Read the model definition and answer for the solid it produces. Units are mm, in the model's axes. Coordinates: 2 decimals unless noted, no trailing zeros. Order: outer loops, then holes, each group sorted by start corner. A loop starts at its lowest first (then second) coordinate and runs counter-clockwise, first axis right, second up. Notation, with made-up numbers: (4.5, 64.5) - (41.5, 64.5) arc R16 cw to (41.5, 83.5) - close; hole circle Ø4 at (6, 50). An arc over 180 degrees is marked (long way). Answer as a JSON object with one key per item and string values. Group by question number.
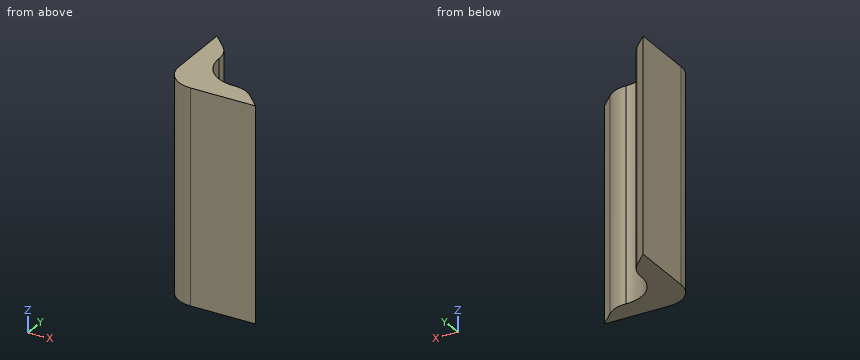
from build123d import *

# Parameters (mm, degrees)
BOSS_EXTRUDE1_DEPTH = 9.525
CHAMFER1_SIZE       = 2
FILLET1_R           = 2.54
FILLET2_R           = 2.54
FILLET3_R           = 3.175


with BuildPart() as part:
    # Sketch1 → Boss-Extrude1 (new, symmetric)
    with BuildSketch(Plane.XY):
        Polygon((0, 0), (8.35, 0), (8.35, 2), (2, 2), (2, 8.35), (0, 8.35), align=None)
    extrude(amount=BOSS_EXTRUDE1_DEPTH, both=True)

    # Chamfer1
    chamfer1_edges = [part.edges().sort_by_distance(p)[0] for p in [
        (8.35, 2, 0),
        (2, 8.35, 0),
    ]]
    chamfer(chamfer1_edges, length=CHAMFER1_SIZE - 0.0001)  # a hair under: the kernel refuses the full size

    # Fillet1
    fillet1_edges = [part.edges().sort_by_distance(p)[0] for p in [
        (6.3501, 2, 0),
        (2, 6.3501, 0),
    ]]
    fillet(fillet1_edges, radius=FILLET1_R)

    # Fillet2
    fillet2_edges = [part.edges().sort_by_distance(p)[0] for p in [
        (0, 0, 0),
    ]]
    fillet(fillet2_edges, radius=FILLET2_R)

    # Fillet3
    fillet3_edges = [part.edges().sort_by_distance(p)[0] for p in [
        (2, 2, 0),
    ]]
    fillet(fillet3_edges, radius=FILLET3_R)


solid = part.part
1. Straight lines are drawn through the part: L1, parallel to Y at x = 5.25, z = 3.75; L2, parallel to X at y = 1.5, z = -8.25; L3, parallel to Y at x = 3, z = -4. For each, find the intervals that lie inside material, in ascending order.
2. Given pin 1 (4 mm diameter, centred on x = 7, z = -4.5, fed in from +Y); pin 2 (1.5 mm diameter, centred on x = 4.5, y = 3, fed in from +Z); pin 3 (1.5 mm diameter, centred on y = 2, z = -7, fed in from +X), each flat-ended and moving along its own axis, determine where each tip first touches the part or whether it passes through.
3. A cutting plane is placed at B-B on y = 6.5. Write down the section's boundary in (x, z) (3 decimals), and give its area (3 significant figures).
4. A cutting plane is placed at C-C on x = 8. Write down the section's boundary in (y, z) (3 decimals), and give its area (3 significant figures).
Derived:
{
 "1": {"L1": "y = 0 to 2", "L2": "x = 0.22 to 6.81", "L3": "y = 0 to 2.86"},
 "2": {"pin 1": "stops at y = 2", "pin 2": "passes through", "pin 3": "stops at x = 7.1"},
 "3": {"outline": "(0, -9.525) - (1.698, -9.525) - (1.698, 9.525) - (0, 9.525) - close", "area": "32.3 mm2"},
 "4": {"outline": "(0, -9.525) - (0.35, -9.525) - (0.35, 9.525) - (0, 9.525) - close", "area": "6.67 mm2"}
}
